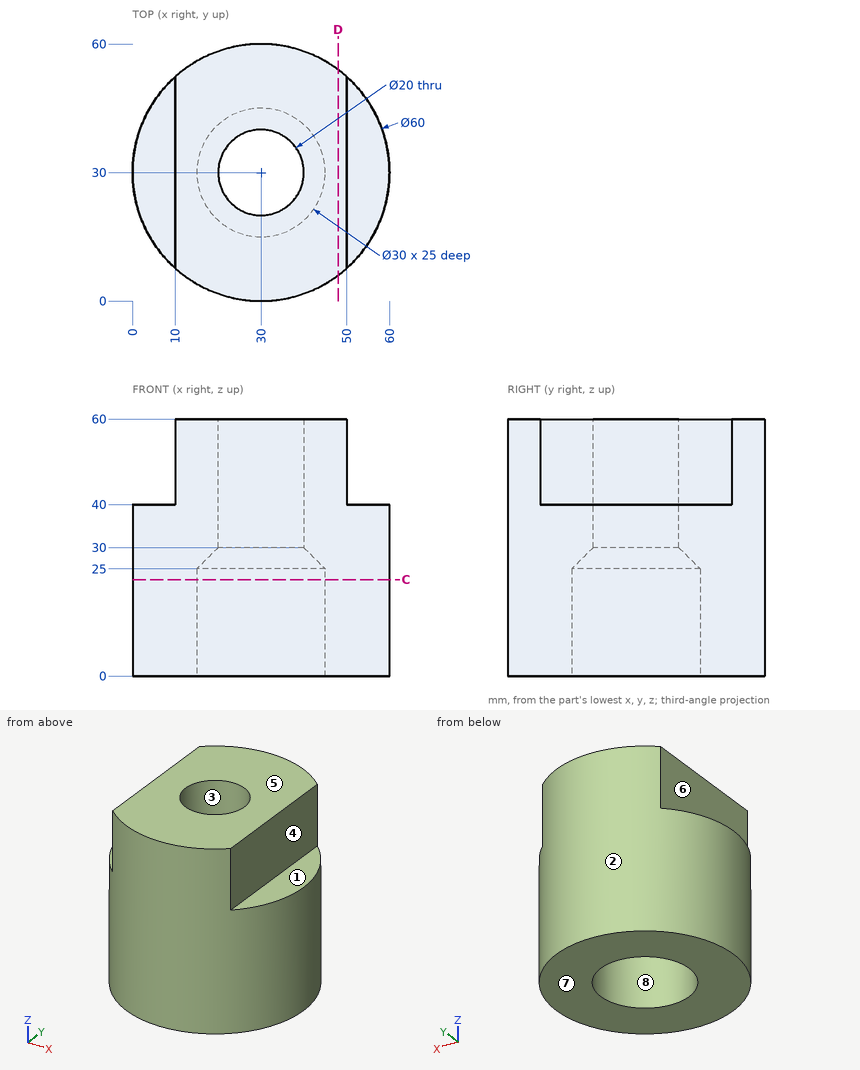
Design review of the part shown in the three views and the two pictorial views. Dimensions are in mm from the part's minimum x, y and z. A direction names the side the tool comes from. Round coordinates to 2 decimals unless told otherwise and drop trailing zeros. Order: outer loops, then holes, each group sorted by start corner. A loop starts at its lowest first (then second) coordinate and runs counter-clockwise, first axis right, second up.
Q1. Wall thickness on line 1 (Y direction, x = 30, z = 10.5); line 2 (Y direction, x = 30, z = 44): over which ranges is each line inside the solid? List them lowest first.
Findings below:
line 1: y = 0 to 15, 45 to 60
line 2: y = 0 to 20, 40 to 60
Q2. We need section C-C, the plane z = 22.5. Give the boundary of the cut face in (x, y), plus the area to 3 significant figures.
Findings below:
outline: circle Ø60 at (30, 30); hole circle Ø30 at (30, 30)
area: 2,120 mm2
Q3. Insertion check: P1, Ø8, axis at x = 44, z = 47, coming from the +Y side; P2, Ø8, axis at x = 15.5, z = 21, coming from the -Y side; P3, Ø2, axis at y = 14.5, z = 15.5, coming from the +X side. Each pin has a flat end and moves straight along its axis. Give the tip position at first contact, or say it passes through.
Findings below:
P1: stops at y = 58.28
P2: stops at y = 1.9
P3: stops at x = 56.26
Q4. We need section D-D, the plane x = 48. Give the boundary of the cut face in (y, z).
Findings below:
outline: (6, 0) - (54, 0) - (54, 60) - (6, 60) - close
Q5. Machinability: for the marked faces 4, 5, 6, 7 and 8, which of the approach directions +Z, -Z, +X, -X, +Y, -Y give a long, thin tool a straight path to every point of the face, cutting with its end or side? Answer none if there is none.
Findings below:
face 4: +Z, +X, +Y, -Y
face 5: +Z, +X, -X, +Y, -Y
face 6: +Z, -X, +Y, -Y
face 7: -Z, +X, -X, +Y, -Y
face 8: -Z
Q6. Mouldability with a two-part tool opening along Y and no side actions: class the marked faces 1, 2 and 3 as pulls with the +Y half, pulls with the -Y half, needs draft (parallel to the pull), parting line crosses it, or undercut.
Findings below:
face 1: needs draft
face 2: parting line crosses it
face 3: undercut
